```python
from build123d import *

# Parameters (mm, degrees)
SKETCH5_R           = 25
BOSS_EXTRUDE1_DEPTH = 1


# Read off the part's stored shape, not the designer's step: Loft-Thin1
with BuildPart() as part:
    # Loft-Thin1 outline → Loft-Thin1 (revolve)
    with BuildSketch(Plane.XY):
        Polygon((38.992217781, 120), (23.992217781, 0), (25, 0), (40, 120), align=None)
    revolve(axis=Axis((0, 0, 0), (0, 1, 0)))

    # Sketch5 → Boss-Extrude1 (add)
    with BuildSketch(Plane.XZ):
        with Locations(Location((0, 0, 0), (0, 0, 270))):
            Circle(SKETCH5_R)
    extrude(amount=BOSS_EXTRUDE1_DEPTH)

    # Sketch6 → Revolve1 (revolve)
    with BuildSketch(Plane.XY, mode=Mode.PRIVATE) as revolve1_sk:
        Polygon((40, 120), (43, 120), (43, 118.5), (42.5, 118.5), (42.5, 119.5), (40, 119.5), (39.9375, 119.5), align=None)
    revolve(revolve1_sk.sketch.rotate(Axis((0, 120, 0), (0, -1, 0)), 90), axis=Axis((0, 120, 0), (0, -1, 0)))


solid = part.part
```
Could you check a few things on this model? Use its own coordinates, in mm. A direction names the side the tool comes from. Coordinates: 2 decimals unless noted, no trailing zeros. Loops run counter-clockwise (first coordinate to the right, second up) from the corner with the lowest first, then second, coordinate; pieces in that order, holes last.
1) Thinking about a two-plate mould opening in X: for faces 1 (the face through (38, 120, -9.4)), 2 (the face through (-42.634, 119.24, -5.598)), 3 (the face through (-12.766, 119.007, 40.537)), which applies, released by +X, released by -X, zero draft, split by the parting line, or undercut?
Reported:
face 1: zero draft
face 2: split by the parting line
face 3: undercut
2) Imagine slicing it at D-D (y = 70). List the corners of the cut face in (x, z) for me.
Reported:
outline: circle Ø67.5 at (0, 0); hole circle Ø65.48 at (0, 0)
3) Will these pins go through, and if not, where does the flat tip stop? pin 1 Ø6 at (y, z) = (17, 19.5) entering from -X; pin 2 Ø5 at (x, y) = (-20, 96) entering from -Z; pin 3 Ø6 at (y, z) = (107.5, -27) entering from +X.
Reported:
pin 1: stops at x = -21.58
pin 2: stops at z = -32.65
pin 3: stops at x = 30.07
4) Which directions (+Z, -Z, +X, -X, +Y, -Y) give clear straight access to the entire face, cutting with the end or side of a thin tool? Please do faces 4 (the face through (0, -1, 0)), 5 (the face through (-13, 119.5, 38)), 6 (the face through (0, 0, 0)).
Reported:
face 4: +Z, -Z, +X, -X, -Y
face 5: -Y
face 6: +Y
5) Imagine slicing it at A-A (x = 0). List the corners of the cut face in (y, z) for me.
Reported:
outline: (-1, -25) - (0, -25) - (119.5, -39.94) - (119.5, -42.5) - (118.5, -42.5) - (118.5, -43) - (120, -43) - (120, -38.99) - (0, -23.99) - (0, 23.99) - (120, 38.99) - (120, 43) - (118.5, 43) - (118.5, 42.5) - (119.5, 42.5) - (119.5, 39.94) - (0, 25) - (-1, 25) - close
6) Imagine slicing it at C-C (y = 43). List the corners of the cut face in (x, z) for me (3 decimals).
Reported:
outline: circle Ø60.75 at (0, 0); hole circle Ø58.734 at (0, 0)
7) Imagine slicing it at B-B (z = 0). List the corners of the cut face in (x, y) for me.
Reported:
outline: (-43, 118.5) - (-42.5, 118.5) - (-42.5, 119.5) - (-39.94, 119.5) - (-25, 0) - (-25, -1) - (25, -1) - (25, 0) - (39.94, 119.5) - (42.5, 119.5) - (42.5, 118.5) - (43, 118.5) - (43, 120) - (38.99, 120) - (23.99, 0) - (-23.99, 0) - (-38.99, 120) - (-43, 120) - close
8) Please list where these lines run through material, in increasing order: line 1 along X through (y, z) = (119.1, 0); line 2 along X through (y, z) = (72, 14.5); line 3 along X through (y, z) = (113.5, -14).
Reported:
line 1: x = -43 to -42.5, -39.89 to -38.88, 38.88 to 39.89, 42.5 to 43
line 2: x = -30.75 to -29.64, 29.64 to 30.75
line 3: x = -36.6 to -35.52, 35.52 to 36.6
